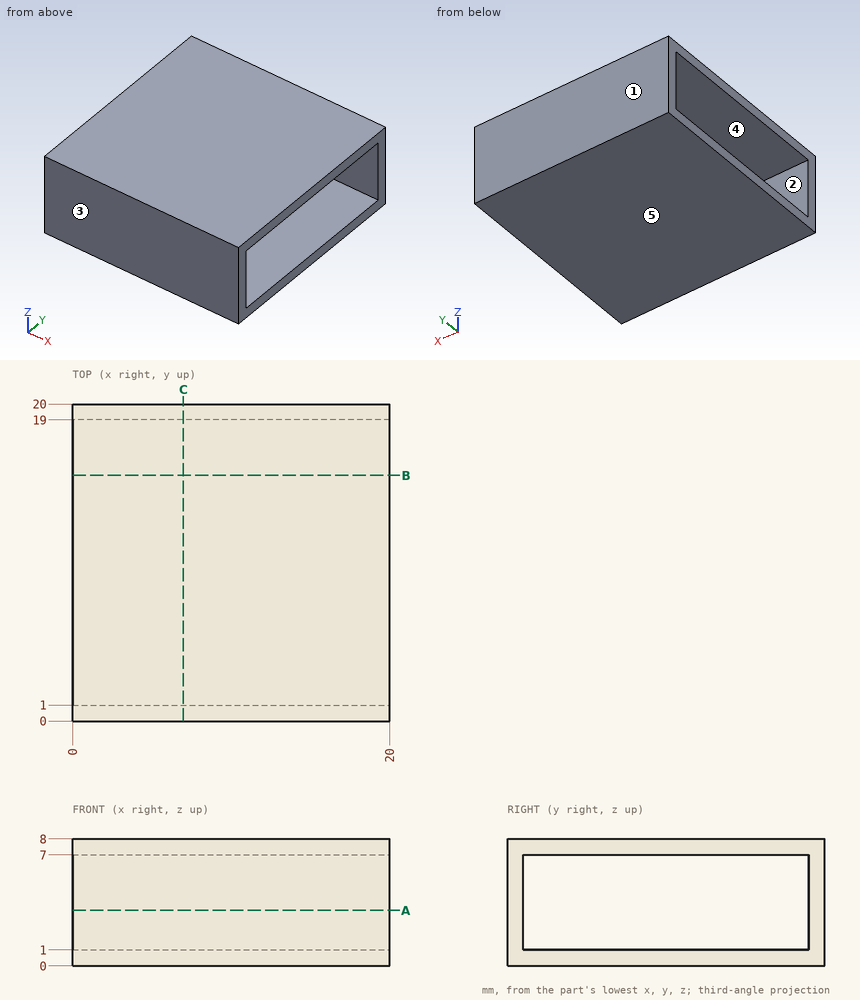
Job drawing, mm, ordinate dimensions from the low corner. One solid piece. A direction names the side the tool comes from. Coordinates: 2 decimals unless noted, no trailing zeros. Write each loop counter-clockwise with the first axis right and the second up, starting at its lowest first coordinate (ties: lowest second). Pieces come first, ordered by that corner, then holes. Notation, with made-up numbers: M -40,41.25 L -11,41.25 A19 ccw -11,74.25 Z; hole C 81,44 d1. An arc over 180 degrees is marked long. Answer as a JSON object with one key per item and string values. Group by question number.
1) Saw through at C-C (x = 7). Write the cut outline in (y, z).
2) Mould opens along Y. For the marked faces 1, 2 and 3 say: +Y half, -Y half, draft (parallel to the pull), parting line (faces both ways), or undercut.
3) Saw through at B-B (y = 15.5). Write the cut outline in (x, z), plus the area to 3 significant figures.
4) Tool access for the marked faces 4 and 5: list every direction of +Z, -Z, +X, -X, +Y, -Y with a clear straight run to the whole face (end or side of a thin tool).
5) Saw through at A-A (z = 3.5). Write the cut outline in (x, y), plus the area to 3 significant figures.
6) Wall check: line 1 (Z direction, x = 8.5, y = 18.75); line 2 (Y direction, x = 16.5, z = 4). Give the ranges that are in metal, low to high. Write a range as from..to.
Values follow:
{
 "1": {"outline": "M 0,0 L 20,0 L 20,8 L 0,8 Z; hole M 1,1 L 19,1 L 19,7 L 1,7 Z"},
 "2": {"face 1": "+Y half", "face 2": "undercut", "face 3": "-Y half"},
 "3": {"outline": "M 0,0 L 20,0 L 20,1 L 0,1 Z; M 0,7 L 20,7 L 20,8 L 0,8 Z", "area": "40.0 mm2"},
 "4": {"face 4": "+X, -X", "face 5": "-Z, +X, -X, +Y, -Y"},
 "5": {"outline": "M 0,0 L 20,0 L 20,1 L 0,1 Z; M 0,19 L 20,19 L 20,20 L 0,20 Z", "area": "40.0 mm2"},
 "6": {"line 1": "z = 0..1, 7..8", "line 2": "y = 0..1, 19..20"}
}
